Design review of the part shown in the three views and the two pictorial views. Dimensions are in mm from the part's minimum x, y and z. A direction names the side the tool comes from. Coordinates: 2 decimals unless noted, no trailing zeros. Write each loop counter-clockwise with the first axis right and the second up, starting at its lowest first coordinate (ties: lowest second). Pieces come first, ordered by that corner, then holes. Notation, with made-up numbers: M 3,58.25 L 61,58.25 A17 cw 61,84.25 Z; hole C 4,-30.5 d7. An arc over 180 degrees is marked long. Answer as a JSON object with one key per item and string values.
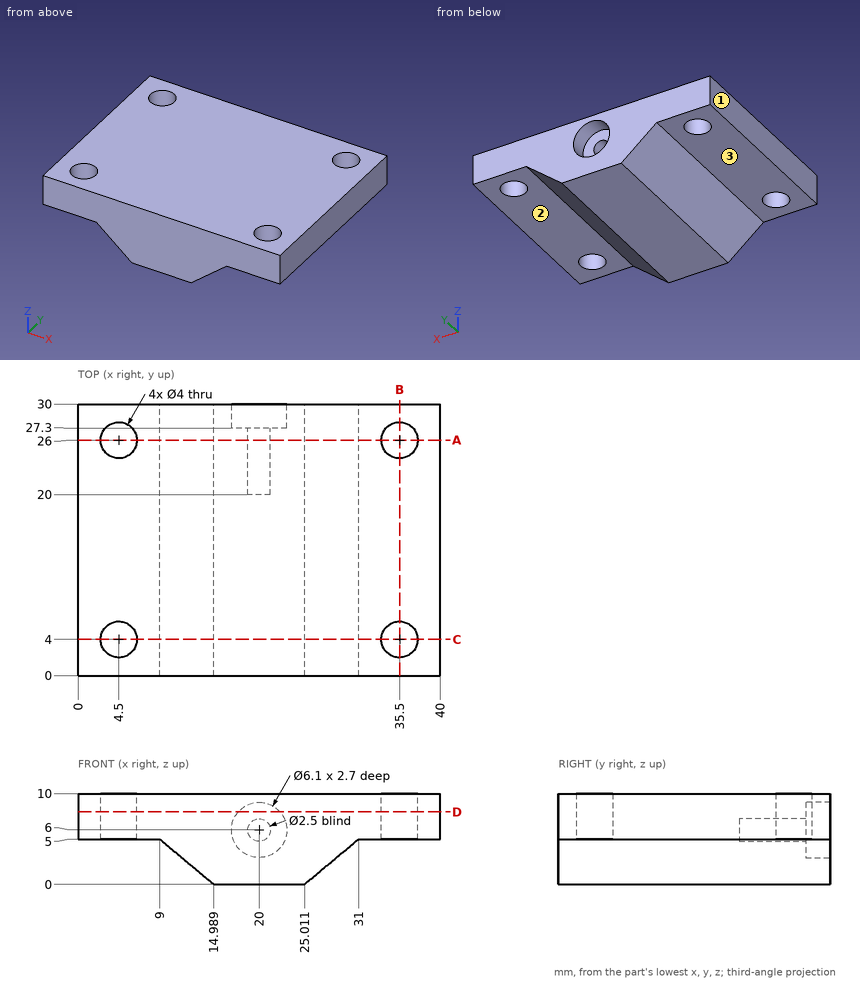
(1) Add section A-A on y = 26. Give the boundary of the cut face in (x, z), and give its area (3 significant figures).
Results list:
{"outline": "M 0,5 L 2.5,5 L 2.5,10 L 0,10 Z; M 6.5,5 L 9,5 L 14.99,0 L 25.01,0 L 31,5 L 33.5,5 L 33.5,10 L 6.5,10 Z; M 37.5,5 L 40,5 L 40,10 L 37.5,10 Z; hole C 20,6 d2.5", "area": "235 mm²"}
(2) Add section D-D on z = 8. Give the boundary of the cut face in (x, y), and give its area (3 significant figures).
Results list:
{"outline": "M 0,0 L 40,0 L 40,30 L 22.3,30 L 22.3,27.3 L 17.7,27.3 L 17.7,30 L 0,30 Z; hole C 4.5,4 d4; hole C 4.5,26 d4; hole C 35.5,4 d4; hole C 35.5,26 d4", "area": "1,140 mm²"}
(3) Add section C-C on y = 4. Give the boundary of the cut face in (x, z).
Results list:
{"outline": "M 0,5 L 2.5,5 L 2.5,10 L 0,10 Z; M 6.5,5 L 9,5 L 14.99,0 L 25.01,0 L 31,5 L 33.5,5 L 33.5,10 L 6.5,10 Z; M 37.5,5 L 40,5 L 40,10 L 37.5,10 Z"}
(4) Wall thickness on line 1 along Y through (x, z) = (35.5, 8.65); line 2 along X through (y, z) = (22.5, 6); line 3 along X through (y, z) = (25.5, 5.5) (1 decimal): over which ranges is each line inside the solid? List them lowest first. Write a range as from..to.
Results list:
{"line 1": "0..2, 6..24, 28..30", "line 2": "0..18.75, 21.25..40", "line 3": "0..2.6, 6.4..18.9, 21.1..33.6, 37.4..40"}
(5) For pin 1 Ø3 at (x, z) = (21, 7.5) entering from +Y; pin 2 Ø2 at (x, z) = (20.5, 6) entering from +Y; pin 3 Ø4.5 at (x, y) = (37, 13) entering from -Z, all flat-tipped, find the tip position at first contact; note any pin that passes through.
Results list:
{"pin 1": "y = 30", "pin 2": "y = 27.3", "pin 3": "z = 5"}
(6) For the marked faces 1, 2 and 3, list the 3-axis set-ups (+Z, -Z, +X, -X, +Y, -Y) from which the entire face can be reached by the end or side of a thin tool; tool diameter is ignored.
Results list:
{"face 1": "+Z, -Z, -X, +Y, -Y", "face 2": "-Z, +X, +Y, -Y", "face 3": "-Z, -X, +Y, -Y"}
(7) Add section B-B on x = 35.5. Give the boundary of the cut face in (y, z), and give its area (3 significant figures).
Results list:
{"outline": "M 0,5 L 2,5 L 2,10 L 0,10 Z; M 6,5 L 24,5 L 24,10 L 6,10 Z; M 28,5 L 30,5 L 30,10 L 28,10 Z", "area": "110 mm²"}
